```python
from build123d import *

# Parameters (mm, degrees)
F0_W     = 25.4
F0_H     = 23.3165774701
F1_DEPTH = 12.7
F3_DEPTH = 25.4
F4_W     = 0.2736736362
F4_H     = 1.0221730918
F4_W_2   = 2.3645318859
F4_W_3   = 0.3372822987
F4_H_2   = 1.0734191164
F4_W_4   = 2.6054769249
F5_DEPTH = 17.78
F7_DEPTH = 25.4


with BuildPart() as f1:
    # F0 (on Front) → F1 (new body, symmetric)
    with BuildSketch(Plane.XZ):
        Rectangle(F0_W, F0_H)
    extrude(amount=F1_DEPTH, both=True)

    # F2 (on face) → F3 (cut)
    with BuildSketch(Plane.XZ.offset(12.7)):
        Polygon((-12.7, 4.811515566), (-3.9780791849, 11.6582887351), (-12.7, 11.6582887351), align=None)
    extrude(amount=-F3_DEPTH, mode=Mode.SUBTRACT)

    # F4 (on face) → F5 (cut)
    with BuildSketch(Plane(origin=(-7.1791973158, 0, 9.1453870251), x_dir=(0.7865883501, 0, 0.6174777466), z_dir=(-0.6174777466, 0, 0.7865883501))):
        with Locations((4.2064599323, 6.4000822604)):
            Rectangle(F4_W, F4_H)
        with Locations((2.8873571713, 6.4000822604)):
            Rectangle(F4_W_2, F4_H)
        with Locations((4.2382642636, 4.0104491636)):
            Rectangle(F4_W_3, F4_H_2)
        with Locations((2.7668846518, 4.0104491636)):
            Rectangle(F4_W_4, F4_H_2)
    extrude(amount=-F5_DEPTH, mode=Mode.SUBTRACT)

    # F6 (on face) → F7 (cut)
    with BuildSketch(Plane.XZ.offset(12.7)):
        Polygon((-21.5201042593, 1.1665492784), (-12.7, 1.1665492784), (-12.7, 4.811515566), (-3.9780791849, 11.6582887351), (-0.8602180751, 11.6582887351), (-0.8602180751, 16.2579510361), (-21.5201042593, 16.2579510361), align=None)
        Polygon((-12.7, 1.1665492784), (-0.8602180751, 1.1665492784), (-0.8602180751, 11.6582887351), (-3.9780791849, 11.6582887351), (-12.7, 4.811515566), align=None)
    extrude(amount=-F7_DEPTH, mode=Mode.SUBTRACT)


solid = f1.part
```
Source: CAD feature listing. Evaluate the final solid. Frame: model axes, mm. A direction names the side the tool comes from. Round coordinates to 2 decimals unless told otherwise and drop trailing zeros. Order: outer loops, then holes, each group sorted by start corner. A loop starts at its lowest first (then second) coordinate and runs counter-clockwise, first axis right, second up. Notation, with made-up numbers: (64, 9.25) -> (85, 9.25) arc R13 cw to (85, 27.25) -> close; hole circle Ø11 at (-19.5, 30.5). An arc over 180 degrees is marked (long way). One line per item, written item: value. Start each with the question number.
Q1. Access query for faces 1 (the flat face through (2.005, 4.003, -0.183)), 2 (the flat face through (-0.86, 0, 6)), 3 (the flat face through (0, 0, -11.658)). Directions: +Z, -Z, +X, -X, +Y, -Y. A direction counts if a zero-diameter tool reaches every point of the face in a straight line with its end or side. Return the directions, or none.
Q2. Section query D-D (x = -1.5). Return the cut outline in (y, z).
Q3. Section query C-C (z = 7.5). Return the cut outline in (x, y) (3 decimals).
Q4. Pin query (flat end, axial travel): pin 1 (8.5 mm diameter, centred on y = -2.5, z = 8, fed in from -X). Return the tip coordinate at first contact, or that it passes through.
Q5. Draft query along Y for faces 4 (the flat face through (6.09, 4.02, -3.04)), 5 (the flat face through (-7, 0, 1.167)), 6 (the flat face through (3, -12.7, -2)), 7 (the flat face through (3, 6.911, 1)). Return one class per face: pulls with the +Y half, pulls with the -Y half, needs draft (parallel to the pull), parting line crosses it, or undercut.
Q6. Section query B-B (y = -10.25). Return the cut outline in (x, z), plus the area to 3 significant figures.
Q7. Section query A-A (x = 1.5). Return the cut outline in (y, z), plus the area to 3 significant figures.
Q8. Material intervals for probe 1 along Y at (x, z) = (0.75, 6); probe 2 along X at (y, z) = (0, 2); probe 3 along Z at (x, y) = (-4.5, -1), sorted ascending.
Findings below:
1. face 1: none
1. face 2: +Z, -X, +Y, -Y
1. face 3: -Z, +X, -X, +Y, -Y
2. outline: (-12.7, -11.66) -> (12.7, -11.66) -> (12.7, 1.17) -> (-12.7, 1.17) -> close
3. outline: (-0.86, -12.7) -> (12.7, -12.7) -> (12.7, 12.7) -> (-0.86, 12.7) -> (-0.86, 6.911) -> (-0.366, 6.911) -> (-0.366, 5.889) -> (-0.86, 5.889) -> (-0.86, 4.547) -> (-0.285, 4.547) -> (-0.285, 3.474) -> (-0.86, 3.474) -> close
4. pin 1: x = -0.86
5. face 4: undercut
5. face 5: needs draft
5. face 6: pulls with the -Y half
5. face 7: undercut
6. outline: (-12.7, -11.66) -> (12.7, -11.66) -> (12.7, 11.66) -> (-0.86, 11.66) -> (-0.86, 1.17) -> (-12.7, 1.17) -> close
6. area: 468 mm²
7. outline: (-12.7, -11.66) -> (12.7, -11.66) -> (12.7, 11.66) -> (-12.7, 11.66) -> close; hole (3.47, 0.46) -> (4.55, 0.46) -> (4.55, 5.23) -> (3.47, 5.23) -> close; hole (5.89, 0.85) -> (6.91, 0.85) -> (6.91, 5.12) -> (5.89, 5.12) -> close
7. area: 583 mm²
8. probe 1: -12.7 to 3.47, 4.55 to 5.89, 6.91 to 12.7
8. probe 2: -0.86 to 12.7
8. probe 3: -11.66 to 1.17
